Part model, mm, in its own coordinate system. A direction names the side the tool comes from. Give positions to 0.01 mm unless a question says otherwise; leave off trailing zeros. Order: outer loops, then holes, each group sorted by start corner. A loop starts at its lowest first (then second) coordinate and runs counter-clockwise, first axis right, second up. Notation, with made-up numbers: (-26.75, -28.75) - (9.25, -28.75) arc R16 cw to (9.25, -1.75) - close; hole circle Ø3 at (-39.5, -1). An arc over 180 degrees is marked (long way). Use one line per item in the form item = value. Start each with the question number.
1. Tool access for faces 5 (the face through (-4, 9.525, 110)), 6 (the face through (-266.7, 0, 56)), 7 (the face through (-38.1, -10, 44)): list every direction of +Z, -Z, +X, -X, +Y, -Y with a clear straight run to the whole face (end or side of a thin tool).
2. Drill centre lines: line 1 (X direction, y = -8.5, z = 79); line 2 (Y direction, x = 35, z = 7.5); line 3 (Z direction, x = -232, y = 8.5) (3 decimals). Where is each one in solid material? Low to high.
3. Band-saw the part on C-C, the plane y = 5. List the corners of the cut face in (x, z) (3 decimals), plus the area to 3 significant figures.
4. Band-saw the part on B-B, the plane z = 51. List the corners of the cut face in (x, y).
5. Pull direction Y, two halves, no side cores. Call faces 1 (the face through (-4, 0, 104.775)), 2 (the face through (-4, -14, 114.3)), 3 (the face through (-4, -9.525, 110)), 4 (the face through (-1, 0, 45)): +Y half, -Y half, draft (parallel to the pull), parting line (faces both ways), or undercut.
6. Pin check, flat tips, straight feed: P1, Ø9.5, axis at x = 18, y = -10.5, coming from the -Z side; P2, Ø8, axis at x = 19.5, z = 14.5, coming from the -Y side. Stop position of each tip, or through.
7. Band-saw the part on A-A, the plane x = -178.5. List the corners of the cut face in (y, z) (3 decimals), plus the area to 3 significant figures.
from build123d import *

# Parameters (mm, degrees)
SKETCH_W        = 533.4
SKETCH_H        = 38.1
PAD_DEPTH       = 114.3
SKETCH001_W     = 762
SKETCH001_H     = 19.05
POCKET_DEPTH    = 9.525
SKETCH003_W     = 76.2
SKETCH003_H     = 88.9
POCKET002_DEPTH = 19.05


with BuildPart() as part:
    # Sketch → Pad (new body)
    with BuildSketch(Plane.XY):
        Rectangle(SKETCH_W, SKETCH_H)
    extrude(amount=PAD_DEPTH)

    # Sketch001 (on Face6 of Pad) → Pocket (cut)
    with BuildSketch(Plane.XY.offset(114.3)):
        Rectangle(SKETCH001_W, SKETCH001_H)
    extrude(amount=-POCKET_DEPTH, mode=Mode.SUBTRACT)

    # Sketch003 → Pocket002 (cut)
    with BuildSketch(Plane.XZ.offset(19.05)):
        with Locations((0, 44.45)):
            Rectangle(SKETCH003_W, SKETCH003_H)
    extrude(amount=-POCKET002_DEPTH, mode=Mode.SUBTRACT)


solid = part.part
From the geometry:
q1.face_5 = +Z, +X, -X
q1.face_6 = +Z, -Z, -X, +Y, -Y
q1.face_7 = -Z, -Y
q2.line_1 = -266.7 to -38.1, 38.1 to 266.7
q2.line_2 = 0 to 19.05
q2.line_3 = 0 to 104.775
q3.outline = (-266.7, 0) - (266.7, 0) - (266.7, 104.775) - (-266.7, 104.775) - close
q3.area = 55,900 mm²
q4.outline = (-266.7, -19.05) - (-38.1, -19.05) - (-38.1, 0) - (38.1, 0) - (38.1, -19.05) - (266.7, -19.05) - (266.7, 19.05) - (-266.7, 19.05) - close
q5.face_1 = undercut
q5.face_2 = draft
q5.face_3 = undercut
q5.face_4 = -Y half
q6.P1 = 88.9
q6.P2 = 0
q7.outline = (-19.05, 0) - (19.05, 0) - (19.05, 114.3) - (9.525, 114.3) - (9.525, 104.775) - (-9.525, 104.775) - (-9.525, 114.3) - (-19.05, 114.3) - close
q7.area = 4,170 mm²
